Source: CAD feature listing. Evaluate the final solid. Frame: model axes, mm. A direction names the side the tool comes from. Give positions to 0.01 mm unless a question says otherwise; leave off trailing zeros. Write each loop counter-clockwise with the first axis right and the second up, starting at its lowest first coordinate (ties: lowest second). Pieces come first, ordered by that corner, then holes.
Autodesk Fusion 360 part; units mm, degrees
sketch "Sketch2" plane through (0, 0, 0) normal (0, 1, 0) x (1, 0, 0)
  circle A0 centre (0, 0) radius 6.75
  circle A1 centre (0, 0) radius 4.25
  line L0 (-3.2862, 6.75) -> (3.2138, 6.75)
  line L1 (3.2138, 6.75) -> (3.2138, 3.75)
  line L2 (3.2138, 3.75) -> (-3.2862, 3.75)
  line L3 (-3.2862, 3.75) -> (-3.2862, 6.75)
  circle A2 centre (0, -4) radius 5.75
  dimension "d1" = 13.5
  dimension "d2" = 8.5
  dimension "d3" = 6.5
  dimension "d4" = 3
  dimension "d5" = 11.5
extrude "Extrude1" add sketch "Sketch2" along normal blind 3.5 contours A0 A1 L1 L2 A2 | A0 A1 A2 | A0 A1 L2 L3 A2 | A1 L2 A2
sketch "Sketch4" plane through (0, 0, 0) normal (1, 0, 0) x (0, 0, -1)
  line L0 (-0.5599, 30.5) -> (0.5599, 30.5)
  line L1 (0.5599, 30.5) -> (0.5599, 13.5)
  line L2 (0.5599, 13.5) -> (-0.5599, 13.5)
  line L3 (-0.5599, 13.5) -> (-0.5599, 30.5)
  line L4 (-0.5599, 30.5) -> (0.5599, 13.5) construction
  line L5 (0.5599, 30.5) -> (-0.5599, 13.5) construction
  line L6 (5.9358, 3.5) -> (-6.75, 3.5)
  line L7 (3.75, 10) -> (1.25, 10)
  line L8 (1.25, 10) -> (1.25, 0)
  line L9 (1.25, 0) -> (3.75, 0)
  line L10 (3.75, 0) -> (3.75, 10)
  line L11 (3.75, 10) -> (0.5599, 13.5)
  line L12 (-0.5599, 13.5) -> (1.25, 10)
  point P0 (0, 22)
  dimension "d8" = 17
  dimension "d9" = 18.5
  dimension "d10" = 2.5
  dimension "d11" = 1.25
  dimension "d12" = 10
extrude "Extrude2" add sketch "Sketch4" along normal mid plane 8
1. Contact query for flat-ended pins moving along their axis: P1, Ø1, axis at x = 2, z = 2, coming from the -Y side; P2, Ø1.5, axis at x = -2, y = 17.5, coming from the +Z side; P3, Ø0.6, axis at y = 2, z = -5.5, coming from the +X side; P4, Ø2.5, axis at x = -1, y = 22, coming from the -Z side. Output: stop coordinate, or through.
2. Cut plane A-A, the plane x = 0. Return the cut outline in (y, z), then the cut area to 3 significant figures.
3. Access query for faces 4 (the flat face through (-3.286, 2, -5)), 5 (the cylindrical face through (-3.38, 1.73, -0.65)), 6 (the flat face through (-4, 15, 0)), 7 (the cylindrical face through (0.09, 1.73, 4.25)). Directions: +Z, -Z, +X, -X, +Y, -Y. A direction counts if a zero-diameter tool reaches every point of the face in a straight line with its end or side. Return the directions, or none.
4. Line query: L1, parallel to Z at x = -1.5, y = 26; L2, parallel to Y at x = -4.5, z = -0.25; L3, parallel to Z at x = 1, y = 9. Output: solid intervals per line, ascending.
5. Cut plane C-C, the plane y = 21. Return the cut outline in (x, z).
6. Cut plane B-B, the plane z = -4.25. Return the cut outline in (x, y), then the cut area to 3 significant figures.
7. Mould query, pull axis Z, two halves, no side actions, for faces 1 (the flat face through (0, 22, -0.56)), 2 (the flat face through (0, 3.5, 5)), 3 (the flat face through (0, 6, -1.25)). Classes: +Z half, -Z half, draft (parallel to the pull), parting line (faces both ways), or undercut.
8. Cut plane D-D, the plane x = -2. Return the cut outline in (y, z), then the cut area to 3 significant figures.
Response values:
1. P1: passes through
1. P2: stops at z = 0.56
1. P3: stops at x = 4.3
1. P4: stops at z = -0.56
2. outline: (0, -3.75) - (10, -3.75) - (13.5, -0.56) - (30.5, -0.56) - (30.5, 0.56) - (13.5, 0.56) - (10, -1.25) - (0, -1.25) - close; (0, 4.25) - (3.5, 4.25) - (3.5, 6.75) - (0, 6.75) - close
2. area: 59.1 mm2
3. face 4: -Z, +Y, -Y
3. face 5: -Y
3. face 6: +Z, -Z, -X, +Y
3. face 7: +Y, -Y
4. L1: z = -0.56 to 0.56
4. L2: y = 0 to 3.5
4. L3: z = -3.75 to -1.25
5. outline: (-4, -0.56) - (4, -0.56) - (4, 0.56) - (-4, 0.56) - close
6. outline: (-5.24, 0) - (-3.29, 0) - (-3.29, 3.5) - (-5.24, 3.5) - close; (3.21, 0) - (5.24, 0) - (5.24, 3.5) - (3.21, 3.5) - close
6. area: 14.0 mm2
7. face 1: -Z half
7. face 2: draft
7. face 3: undercut
8. outline: (0, -3.75) - (10, -3.75) - (13.5, -0.56) - (30.5, -0.56) - (30.5, 0.56) - (13.5, 0.56) - (10, -1.25) - (0, -1.25) - close; (0, 3.75) - (3.5, 3.75) - (3.5, 6.45) - (0, 6.45) - close
8. area: 59.8 mm2
